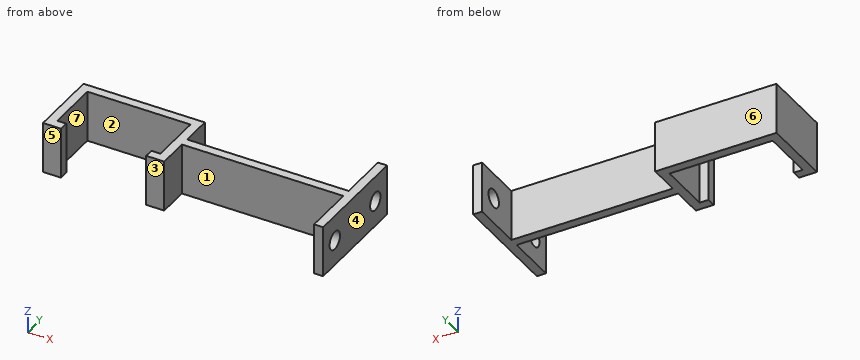
```python
from build123d import *

# Parameters (mm, degrees)
BOSS_EXTRU_1_DEPTH      = 11.3
ESQUISSE2_W             = 8.8
ESQUISSE2_H             = 11.3
BOSS_EXTRU_2_DEPTH      = 1
ESQUISSE8_W             = 11.3
ESQUISSE8_H             = 1
BOSS_EXTRU_5_DEPTH      = 10
ESQUISSE9_W             = 2
ESQUISSE9_H             = 11.3
BOSS_EXTRU_6_DEPTH      = 7.8
ESQUISSE10_W            = 11.3
ESQUISSE10_H            = 2
BOSS_EXTRU_7_DEPTH      = 36.7
ESQUISSE11_W            = 2
ESQUISSE11_H            = 11.3
BOSS_EXTRU_8_DEPTH      = 11.3
ESQUISSE12_W            = 2
ESQUISSE12_H            = 11.3
BOSS_EXTRU_9_DEPTH      = 11.3
BOSS_EXTRU_10_DEPTH     = 11.3
ESQUISSE14_W            = 1
ESQUISSE14_H            = 11.3
BOSS_EXTRU_11_DEPTH     = 5.8
ESQUISSE16_W            = 11.3
ESQUISSE16_H            = 6.8
ENL_V_MAT_EXTRU_1_DEPTH = 1
ESQUISSE19_R            = 2
ENL_V_MAT_EXTRU_3_DEPTH = 10
ESQUISSE22_W            = 4
ESQUISSE22_H            = 1
BOSS_EXTRU_12_DEPTH     = 11.3


with BuildPart() as part:
    # Esquisse1 → Boss.-Extru.1 (new body)
    with BuildSketch(Plane.XY):
        Polygon((-21.8, 1), (-21.8, 0), (-24.8, 0), (-24.8, 13.6), (0, 13.6), (0, 0), (-3, 0), (-3, 1), (-1, 1), (-1, 12.6), (-23.8, 12.6), (-23.8, 1), align=None)
    extrude(amount=BOSS_EXTRU_1_DEPTH)

    # Esquisse2 → Boss.-Extru.2 (add)
    with BuildSketch(Plane(origin=(0, 13.6, 0), x_dir=(1, 0, 0), z_dir=(0, 1, 0))):
        with Locations((-12.4, -5.65)):
            Rectangle(ESQUISSE2_W, ESQUISSE2_H)
    extrude(amount=BOSS_EXTRU_2_DEPTH)

    # Esquisse8 → Boss.-Extru.5 (add)
    with BuildSketch(Plane(origin=(-8, 0, 0), x_dir=(0, 0, -1), z_dir=(1, 0, 0))):
        with Locations((-5.65, 14.1)):
            Rectangle(ESQUISSE8_W, ESQUISSE8_H)
    extrude(amount=BOSS_EXTRU_5_DEPTH)

    # Esquisse9 → Boss.-Extru.6 (add)
    with BuildSketch(Plane.XZ.offset(-13.6)):
        with Locations((1, 5.65)):
            Rectangle(ESQUISSE9_W, ESQUISSE9_H)
    extrude(amount=BOSS_EXTRU_6_DEPTH)

    # Esquisse10 → Boss.-Extru.7 (add)
    with BuildSketch(Plane(origin=(2, 0, 0), x_dir=(0, 0, -1), z_dir=(1, 0, 0))):
        with Locations((-5.65, 6.8)):
            Rectangle(ESQUISSE10_W, ESQUISSE10_H)
    extrude(amount=BOSS_EXTRU_7_DEPTH)

    # Esquisse11 → Boss.-Extru.8 (add)
    with BuildSketch(Plane.XZ.offset(-5.8)):
        with Locations((37.7, 5.65)):
            Rectangle(ESQUISSE11_W, ESQUISSE11_H)
    extrude(amount=BOSS_EXTRU_8_DEPTH)

    # Esquisse12 → Boss.-Extru.9 (add)
    with BuildSketch(Plane(origin=(0, 7.8, 0), x_dir=(1, 0, 0), z_dir=(0, 1, 0))):
        with Locations((37.7, -5.65)):
            Rectangle(ESQUISSE12_W, ESQUISSE12_H)
    extrude(amount=BOSS_EXTRU_9_DEPTH)

    # Esquisse13 → Boss.-Extru.10 (add)
    with BuildSketch(Plane.XY.offset(11.3)):
        Polygon((-16.8, 14.6), (-25.8, 14.6), (-25.8, 0), (-24.8, 0), (-24.8, 13.6), (-16.8, 13.6), align=None)
    extrude(amount=-BOSS_EXTRU_10_DEPTH)

    # Esquisse14 → Boss.-Extru.11 (add)
    with BuildSketch(Plane.XZ.offset(-5.8)):
        with Locations((0.5, 5.65)):
            Rectangle(ESQUISSE14_W, ESQUISSE14_H)
    extrude(amount=BOSS_EXTRU_11_DEPTH)

    # Esquisse16 → Enlèv. mat.-Extru.1 (cut)
    with BuildSketch(Plane(origin=(2, 0, 0), x_dir=(0, 0, -1), z_dir=(1, 0, 0))):
        with Locations((-5.65, 11.2)):
            Rectangle(ESQUISSE16_W, ESQUISSE16_H)
    extrude(amount=-ENL_V_MAT_EXTRU_1_DEPTH, mode=Mode.SUBTRACT)

    # Esquisse19 → Enlèv. mat.-Extru.3 (cut)
    with BuildSketch(Plane(origin=(38.7, 0, 0), x_dir=(0, 0, -1), z_dir=(1, 0, 0))):
        with Locations((-5.65, 14.6)):
            Circle(ESQUISSE19_R)
        with Locations((-5.65, -1)):
            Circle(ESQUISSE19_R)
    extrude(amount=-ENL_V_MAT_EXTRU_3_DEPTH, mode=Mode.SUBTRACT)

    # Esquisse22 → Boss.-Extru.12 (add)
    with BuildSketch(Plane.XY.offset(11.3)):
        with Locations((-23.8, -0.5)):
            Rectangle(ESQUISSE22_W, ESQUISSE22_H)
        with Locations((-1, -0.5)):
            Rectangle(ESQUISSE22_W, ESQUISSE22_H)
    extrude(amount=-BOSS_EXTRU_12_DEPTH)


solid = part.part
```
Work out the finished part from the listing and answer in its coordinate system (mm). Face numbers are marked on the shaded views. A direction names the side the tool comes from. Round coordinates to 2 decimals unless told otherwise and drop trailing zeros. Write each loop counter-clockwise with the first axis right and the second up, starting at its lowest first coordinate (ties: lowest second). Pieces come first, ordered by that corner, then holes. Notation, with made-up numbers: (67, -10.5) - (97, -10.5) arc R24 ccw to (97, 7.5) - close; hole circle Ø9 at (-19, 81.5). An arc over 180 degrees is marked (long way). Return JSON: item names as keys, results as strings. Group by question number.
Q1. The part is cut by section D-D on y = -3.75. Write down the section's boundary in (x, z), then the cut area to 3 significant figures.
Q2. Find the intervals of material crossed by L1, parallel to Y at x = 37.95, z = 5.65; L2, parallel to X at y = 0, z = 10.75; L3, parallel to X at y = 11, z = 7, in increasing order.
Q3. The part is cut by section A-A on z = 5.65. Write down the section's boundary in (x, y).
Q4. The part is cut by section C-C on z = 9. Write down the section's boundary in (x, y), then the cut area to 3 significant figures.
Q5. For the marked faces 5, 6 and 7, determine the directions among +Z, -Z, +X, -X, +Y, -Y from which every point of the face is accessible in a straight line to the end or side of a thin tool.
Q6. The mould has two halves that part along X. Classify the marked faces 1, 2, 3 and 4: released by +X, released by -X, zero draft, split by the parting line, or undercut.
Q7. Each of these flat-tipped pins is pushed along its axis until it touches: pin 1 Ø5.5 at (x, z) = (24, 4) entering from -Y; pin 2 Ø1 at (x, z) = (-1.5, 8) entering from +Y; pin 3 Ø3 at (x, z) = (-23, 3) entering from -Y. Where does it stop, or does it pass through?
Q8. The part is cut by section B-B on y = 13.5. Write down the section's boundary in (x, z), then the cut area to 3 significant figures.
Solved:
{
 "1": {"outline": "(36.7, 0) - (38.7, 0) - (38.7, 11.3) - (36.7, 11.3) - close", "area": "22.6 mm²"},
 "2": {"L1": "-5.5 to -3, 1 to 12.6, 16.6 to 19.1", "L2": "-25.8 to -21.8, -3 to 1, 36.7 to 38.7", "L3": "-25.8 to -23.8, -1 to 1, 36.7 to 38.7"},
 "3": {"outline": "(-25.8, -1) - (-21.8, -1) - (-21.8, 1) - (-23.8, 1) - (-23.8, 12.6) - (-1, 12.6) - (-1, 1) - (-3, 1) - (-3, -1) - (1, -1) - (1, 5.8) - (36.7, 5.8) - (36.7, 1) - (38.7, 1) - (38.7, 12.6) - (36.7, 12.6) - (36.7, 7.8) - (1, 7.8) - (1, 14.6) - (-25.8, 14.6) - close; (36.7, -5.5) - (38.7, -5.5) - (38.7, -3) - (36.7, -3) - close; (36.7, 16.6) - (38.7, 16.6) - (38.7, 19.1) - (36.7, 19.1) - close"},
 "4": {"outline": "(-25.8, -1) - (-21.8, -1) - (-21.8, 1) - (-23.8, 1) - (-23.8, 12.6) - (-1, 12.6) - (-1, 1) - (-3, 1) - (-3, -1) - (1, -1) - (1, 5.8) - (36.7, 5.8) - (36.7, -5.5) - (38.7, -5.5) - (38.7, 19.1) - (36.7, 19.1) - (36.7, 7.8) - (1, 7.8) - (1, 14.6) - (-25.8, 14.6) - close", "area": "237 mm²"},
 "5": {"face 5": "+Z, -Z, -X, -Y", "face 6": "+Z, -Z, -X, +Y", "face 7": "+Z, -Z"},
 "6": {"face 1": "undercut", "face 2": "undercut", "face 3": "zero draft", "face 4": "released by +X"},
 "7": {"pin 1": "y = 5.8", "pin 2": "y = 14.6", "pin 3": "y = -1"},
 "8": {"outline": "(-25.8, 0) - (1, 0) - (1, 11.3) - (-25.8, 11.3) - close; (36.7, 0) - (38.7, 0) - (38.7, 3.98) - (36.7, 3.98) - close; (36.7, 7.32) - (38.7, 7.32) - (38.7, 11.3) - (36.7, 11.3) - close", "area": "319 mm²"}
}
